from build123d import *

# Parameters (mm, degrees)
EXTRUDE_1_DEPTH = 24
FILLET_1_R      = 1
SKETCH_870_R    = 0.55
EXTRUDE_2_DEPTH = 3.5


with BuildPart() as part:
    # Эскиз1 → Бобышка-Вытянуть1 (new body)
    with BuildSketch(Plane(origin=(0, 0, 0), x_dir=(1, 0, 0), z_dir=(0, 1, 0))):
        with BuildLine():
            Line((-25.2, 13.6), (25.2, 13.6))
            ThreePointArc((25.2, 13.6), (25.907106781, 13.307106781), (26.2, 12.6))
            Line((26.2, 12.6), (26.2, -12.6))
            ThreePointArc((26.2, -12.6), (25.907106781, -13.307106781), (25.2, -13.6))
            Line((25.2, -13.6), (-25.2, -13.6))
            ThreePointArc((-25.2, -13.6), (-25.907106781, -13.307106781), (-26.2, -12.6))
            Line((-26.2, -12.6), (-26.2, 12.6))
            ThreePointArc((-26.2, 12.6), (-25.907106781, 13.307106781), (-25.2, 13.6))
        make_face()
    extrude(amount=EXTRUDE_1_DEPTH)

    # Скругление1
    fillet_1_edges = [part.edges().sort_by_distance(p)[0] for p in [
        (-25.907106781, 24, -13.307106781),
        (-26.2, 24, 0),
        (-25.907106781, 24, 13.307106781),
        (0, 24, 13.6),
        (25.907106781, 24, 13.307106781),
        (26.2, 24, 0),
        (25.907106781, 24, -13.307106781),
        (0, 24, -13.6),
    ]]
    fillet(fillet_1_edges, radius=FILLET_1_R)

    # Sketch 870 → Бобышка-Вытянуть2 (add)
    with BuildSketch(Plane.XZ):
        with Locations((-22.8, 10.4)):
            Circle(SKETCH_870_R)
        with Locations((-22.8, -10.4)):
            Circle(SKETCH_870_R)
        with Locations((22.2, 10.4)):
            Circle(SKETCH_870_R)
        with Locations((22.2, 2.4)):
            Circle(SKETCH_870_R)
    extrude(amount=EXTRUDE_2_DEPTH)


solid = part.part
Verification items for the finished model (mm, model axes). A direction names the side the tool comes from. Give positions to 0.01 mm unless a question says otherwise; leave off trailing zeros. Write each loop counter-clockwise with the first axis right and the second up, starting at its lowest first coordinate (ties: lowest second). Pieces come first, ordered by that corner, then holes. Notation, with made-up numbers: (72.25, -17) -> (113.25, -17) arc R17 ccw to (113.25, 6) -> close; hole circle Ø2 at (26.25, -27). An arc over 180 degrees is marked (long way). Use CSV: the item, a comma, the result in double quotes.
(1) Sectioned sample at C-C (z = -7.25). Record the cut outline in (x, y).
Derived:
outline,"(-26.2, 0) -> (26.2, 0) -> (26.2, 23) arc R1 ccw to (25.2, 24) -> (-25.2, 24) arc R1 ccw to (-26.2, 23) -> close"
(2) Go/stop test with a flat-tipped pin: pin 1 (8 mm diameter, centred on x = -2, z = -5.5, fed in from -Y). Record where the tip stops, or that it passes through.
Derived:
pin 1,"stops at y = 0"
(3) Set-up check for faces 5 (the flat face through (22.2, -3.5, 10.4)), 6 (the cylindrical face through (-22.872, -1.726, -9.855)): record each of +Z, -Z, +X, -X, +Y, -Y from which the full face is reachable in a straight line by a thin tool's end or side.
Derived:
face 5,"+Z, -Z, +X, -X, -Y"
face 6,"-Y"
(4) Sectioned sample at D-D (x = 14). Record the cut outline in (y, z).
Derived:
outline,"(0, -13.6) -> (23, -13.6) arc R1 ccw to (24, -12.6) -> (24, 12.6) arc R1 ccw to (23, 13.6) -> (0, 13.6) -> close"
(5) Release check for a two-part mould opening along Z. For faces 1 (the cylindrical face through (-22.919, -1.726, 9.863)), 2 (the cylindrical face through (0.353, 23.699, -13.315)), 3 (the cylindrical face through (-25.915, 23.699, -0.176)), 4 (the cylindrical face through (-25.899, 11.339, 13.315)) record: +Z half, -Z half, draft (parallel to the pull), parting line (faces both ways), or undercut.
Derived:
face 1,"undercut"
face 2,"-Z half"
face 3,"draft"
face 4,"+Z half"
(6) Material ranges on L1, parallel to X at y = -1.75, z = 10.5; L2, parallel to Y at x = 4.5, z = 0.5; L3, parallel to X at y = 15.5, z = 12.75, recorded low to high.
Derived:
L1,"x = -23.34 to -22.26, 21.66 to 22.74"
L2,"y = 0 to 24"
L3,"x = -26.19 to 26.19"
(7) Sectioned sample at B-B (x = -22.8). Record the cut outline in (y, z).
Derived:
outline,"(-3.5, -10.95) -> (0, -10.95) -> (0, -13.6) -> (23, -13.6) arc R1 ccw to (24, -12.6) -> (24, 12.6) arc R1 ccw to (23, 13.6) -> (0, 13.6) -> (0, 10.95) -> (-3.5, 10.95) -> (-3.5, 9.85) -> (0, 9.85) -> (0, -9.85) -> (-3.5, -9.85) -> close"
(8) Sectioned sample at A-A (z = -10.4). Record the cut outline in (x, y).
Derived:
outline,"(-26.2, 0) -> (-23.35, 0) -> (-23.35, -3.5) -> (-22.25, -3.5) -> (-22.25, 0) -> (26.2, 0) -> (26.2, 23) arc R1 ccw to (25.2, 24) -> (-25.2, 24) arc R1 ccw to (-26.2, 23) -> close"
